Autodesk Inventor part; units mm, degrees
ref_plane "YZ Plane" through (0, 0, 0) normal (1, 0, 0) x (0, 1, 0)
ref_plane "XZ Plane" through (0, 0, 0) normal (0, 1, 0) x (-1, 0, 0)
ref_plane "XY Plane" through (0, 0, 0) normal (0, 0, 1) x (1, 0, 0)
sketch "Esquisse1" plane through (0, 0, 0) normal (0, 0, 1) x (1, 0, 0)
  circle A0 centre (0, 0) radius 2
  circle A1 centre (0, 0) radius 6.5
  dimension "d0" = 4
  dimension "d1" = 13
extrude "Extrusion1" add sketch "Esquisse1" along normal blind 5
sketch "Esquisse2" plane through (0, 0, 5) normal (0, 0, 1) x (1, 0, 0)
  circle A0 centre (0, 0) radius 2
  circle A1 centre (0, 0) radius 6.5
  circle A2 centre (0, 0) radius 2.75
  circle A3 centre (0, 0) radius 5.75
  dimension "d4" = 11.5
  dimension "d5" = 13
  dimension "d6" = 4
  dimension "d7" = 5.5
extrude "Extrusion2" cut sketch "Esquisse2" against normal blind 0.5 contours A3
sketch "Esquisse3" plane through (0, 0, 0) normal (0, 0, -1) x (-1, 0, 0)
  circle A0 centre (0, 0) radius 2
  circle A1 centre (0, 0) radius 6.5
  circle A2 centre (0, 0) radius 2.75
  circle A3 centre (0, 0) radius 5.75
  dimension "d12" = 11.5
  dimension "d13" = 13
  dimension "d14" = 4
  dimension "d15" = 5.5
extrude "Extrusion3" cut sketch "Esquisse3" against normal blind 0.5 contours A3
properties part number "Roulement" material "Acier"
CAD build for the part. Positions are in the model's coordinates, mm. A direction names the side the tool comes from. Round coordinates to 2 decimals unless told otherwise and drop trailing zeros. Loops run counter-clockwise (first coordinate to the right, second up) from the corner with the lowest first, then second, coordinate; pieces in that order, holes last. Notation, with made-up numbers: (70, 61.25) - (104, 61.25) arc R21 ccw to (104, 93.25) - close; hole circle Ø11 at (12.25, 27). An arc over 180 degrees is marked (long way). Put each result on its own line as item: value.
1. 3-axis set-ups, long thin cutter, end or side, ignore diameter. For faces 1 (the cylindrical face through (0, 2, 2)), 2 (the cylindrical face through (0.75, 5.7, 0.25)), 3 (the cylindrical face through (-0.596, -2.685, 4.754)): which of +Z, -Z, +X, -X, +Y, -Y reach the whole face in a straight line?
Geometry check:
face 1: +Z, -Z
face 2: -Z
face 3: +Z
2. Wall check: line 1 (Y direction, x = 0, z = 4.65); line 2 (Y direction, x = 0, z = 1.2); line 3 (Z direction, x = -4, y = 2). Give the ranges that are in metal, low to high.
Geometry check:
line 1: -6.5 to -5.75, -2.75 to -2, 2 to 2.75, 5.75 to 6.5
line 2: -6.5 to -2, 2 to 6.5
line 3: 0.5 to 4.5
3. Slice it at A-A on x = 0. List the corners of the cut face in (y, z), and give its area (3 significant figures).
Geometry check:
outline: (-6.5, 0) - (-5.75, 0) - (-5.75, 0.5) - (-2.75, 0.5) - (-2.75, 0) - (-2, 0) - (-2, 5) - (-2.75, 5) - (-2.75, 4.5) - (-5.75, 4.5) - (-5.75, 5) - (-6.5, 5) - close; (2, 0) - (2.75, 0) - (2.75, 0.5) - (5.75, 0.5) - (5.75, 0) - (6.5, 0) - (6.5, 5) - (5.75, 5) - (5.75, 4.5) - (2.75, 4.5) - (2.75, 5) - (2, 5) - close
area: 39.0 mm²
4. Pin check, flat tips, straight feed: P1, Ø2.5, axis at x = 0, y = 0, coming from the +Z side; P2, Ø1.5, axis at x = -1, y = -3.5, coming from the -Z side; P3, Ø3, axis at x = 3, z = 3, coming from the +Y side. Stop position of each tip, or through.
Geometry check:
P1: through
P2: z = 0.5
P3: y = 6.32
5. Slice it at D-D on y = -3. List the corners of the cut face in (x, z).
Geometry check:
outline: (-5.77, 0) - (-4.91, 0) - (-4.91, 0.5) - (4.91, 0.5) - (4.91, 0) - (5.77, 0) - (5.77, 5) - (4.91, 5) - (4.91, 4.5) - (-4.91, 4.5) - (-4.91, 5) - (-5.77, 5) - close
6. Slice it at C-C on z = 0.9. List the corners of the cut face in (x, y), and give its area (3 significant figures).
Geometry check:
outline: circle Ø13 at (0, 0); hole circle Ø4 at (0, 0)
area: 120 mm²
7. Two-plate mould, pull along Y, no slides. Class faces 4 (the cylindrical face through (0.596, -2.685, 0.246)), 5 (the flat face through (0, -6, 5)), 6 (the cylindrical face through (-5.158, 3.955, 2.465)): released by +Y, released by -Y, zero draft, split by the parting line, or undercut.
Geometry check:
face 4: undercut
face 5: zero draft
face 6: split by the parting line
